The listing builds one solid part. Answer for the finished solid, in the listing's coordinates (mm). Round coordinates to 2 decimals unless told otherwise and drop trailing zeros. Write each loop counter-clockwise with the first axis right and the second up, starting at its lowest first coordinate (ties: lowest second). Pieces come first, ordered by that corner, then holes. Notation, with made-up numbers: (48, 79) - (59, 79) arc R23 cw to (59, 100) - close; hole circle Ø6 at (55, 46). An arc over 180 degrees is marked (long way). Return JSON: item names as keys, results as strings. Group by question number.
(1) Each of these flat-tipped pins is pushed along its axis until it touches: pin 1 (5 mm diameter, centred on x = -32.81, z = -52.81, fed in from -Y); pin 2 (3 mm diameter, centred on x = 33.5, z = 12.5, fed in from +Y); pin 3 (4 mm diameter, centred on x = 25, y = 575, fed in from +Z). Where does it stop, or does it pass through?
(2) Find the intervals of material crossed by line 1 along Y through (x, z) = (-1, -52.5); line 2 along Y through (x, z) = (-5, 2.5); line 3 along Z through (x, y) = (27.5, 52.5), in increasing order. Write a range as [from, to].
(3) Section A-A, the plane y = 30 is taken. Write down the section's boundary in (x, z), then the cut area to 3 significant figures.
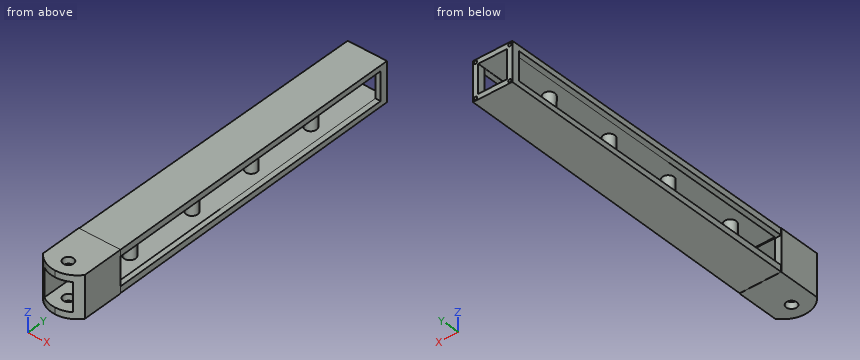
```python
from build123d import *

# Parameters (mm, degrees)
SKETCH1_W               = 80
SKETCH1_H               = 80
BOSS_EXTRUDE1_DEPTH     = 700
BOSS_EXTRUDE1_TAPER     = 0.2
SHELL2_T                = -10
SKETCH2_R               = 3
CUT_EXTRUDE1_DEPTH      = 10
CUT_EXTRUDE2_DEPTH      = 704.704483544
CUT_EXTRUDE2_DEPTH_BACK = 704.704483544
SKETCH4_W               = 55.112936398
SKETCH4_H               = 55.112936398
SKETCH8_W               = 80
SKETCH8_H               = 80
SKETCH8_W_2             = 55.112936398
SKETCH8_H_2             = 55.112936398
BOSS_EXTRUDE3_DEPTH     = 100
CUT_EXTRUDE4_DEPTH      = 706.691150691
CUT_EXTRUDE4_DEPTH_BACK = 706.691150691
SKETCH9_R               = 10
CUT_EXTRUDE5_DEPTH      = 706.691150691
CUT_EXTRUDE5_DEPTH_BACK = 706.691150691
CUT_EXTRUDE6_DEPTH      = 707.968504527
CUT_EXTRUDE6_DEPTH_BACK = 707.968504527
SKETCH13_W              = 54.721685152
SKETCH13_H              = 585.463174199
SKETCH14_R              = 11
BOSS_EXTRUDE4_DEPTH     = 68


with BuildPart() as part:
    # Sketch1 → Boss-Extrude1 (new body)
    with BuildSketch(Plane(origin=(0, 0, 0), x_dir=(1, 0, 0), z_dir=(0, 1, 0))):
        with Locations((0, 20)):
            Rectangle(SKETCH1_W, SKETCH1_H)
    extrude(amount=BOSS_EXTRUDE1_DEPTH, taper=BOSS_EXTRUDE1_TAPER)

    # Shell2
    shell2_openings = [part.faces().sort_by_distance(p)[0] for p in [
        (0, 700, -20),
    ]]
    offset(amount=SHELL2_T, openings=shell2_openings, kind=Kind.INTERSECTION)

    # Sketch2 → Cut-Extrude1 (cut)
    with BuildSketch(Plane(origin=(0, 700, 0), x_dir=(1, 0, 0), z_dir=(0, 1, 0))):
        with Locations(Location((-32.80796506, 52.80796506, 0), (0, 0, 270))):
            Circle(SKETCH2_R)
        with Locations(Location((32.80796506, 52.80796506, 0), (0, 0, 90))):
            Circle(SKETCH2_R)
        with Locations(Location((32.80796506, -12.80796506, 0), (0, 0, 270))):
            Circle(SKETCH2_R)
        with Locations(Location((-32.80796506, -12.80796506, 0), (0, 0, 90))):
            Circle(SKETCH2_R)
    extrude(amount=-CUT_EXTRUDE1_DEPTH, mode=Mode.SUBTRACT)

    # Sketch4 → Cut-Extrude2 (cut, two sides: drawn at the far end of the back side and taken through both)
    with BuildSketch(Plane(origin=(0, 700, 0), x_dir=(1, 0, 0), z_dir=(0, 1, 0)).offset(-CUT_EXTRUDE2_DEPTH_BACK)):
        with Locations((0, 20)):
            Rectangle(SKETCH4_W, SKETCH4_H)
    extrude(amount=CUT_EXTRUDE2_DEPTH + CUT_EXTRUDE2_DEPTH_BACK, mode=Mode.SUBTRACT)

    # Sketch8 → Boss-Extrude3 (add)
    with BuildSketch(Plane.XZ):
        with Locations((0, -20)):
            Rectangle(SKETCH8_W, SKETCH8_H)
        with Locations((0, -20)):
            Rectangle(SKETCH8_W_2, SKETCH8_H_2, mode=Mode.SUBTRACT)
    extrude(amount=-BOSS_EXTRUDE3_DEPTH)

    # Sketch9 → Cut-Extrude4 (cut, two sides: drawn at the far end of the back side and taken through both)
    with BuildSketch(Plane.XY.offset(20).offset(-CUT_EXTRUDE4_DEPTH_BACK)):
        with Locations((0, 30)):
            Circle(SKETCH9_R)
    extrude(amount=CUT_EXTRUDE4_DEPTH + CUT_EXTRUDE4_DEPTH_BACK, mode=Mode.SUBTRACT)

    # Sketch10 → Cut-Extrude5 (cut, two sides: drawn at the far end of the back side and taken through both)
    with BuildSketch(Plane.XY.offset(20).offset(-CUT_EXTRUDE5_DEPTH_BACK)):
        with BuildLine():
            Line((-40, 0), (-1.42e-07, 0))
            ThreePointArc((-1.42e-07, 0), (-22.333063671, 5.242902067), (-40, 19.876189785))
            Line((-40, 19.876189785), (-40, 0))
        make_face()
        with BuildLine():
            Line((-1.42e-07, 0), (40, 0))
            Line((40, 0), (40, 19.876189785))
            ThreePointArc((40, 19.876189785), (22.333063544, 5.242902004), (-1.42e-07, 0))
        make_face()
    extrude(amount=CUT_EXTRUDE5_DEPTH + CUT_EXTRUDE5_DEPTH_BACK, mode=Mode.SUBTRACT)

    # Sketch13 → Cut-Extrude6 (cut, two sides: drawn at the far end of the back side and taken through both)
    with BuildSketch(Plane(origin=(39.999512614, 0.139625206, 0), x_dir=(0, 0, -1), z_dir=(0.9999939076577905, 0.0034906514152237404, 0)).offset(-CUT_EXTRUDE6_DEPTH_BACK)):
        with Locations((20, 392.592570281)):
            Rectangle(SKETCH13_W, SKETCH13_H)
    extrude(amount=CUT_EXTRUDE6_DEPTH + CUT_EXTRUDE6_DEPTH_BACK, mode=Mode.SUBTRACT)

    # Sketch14 → Boss-Extrude4 (add)
    with BuildSketch(Plane(origin=(0, 0.209437809, -59.999268921), x_dir=(-1, 0, 0), z_dir=(0, 0.0034906514152237404, -0.9999939076577905))):
        with Locations(Location((0, 167.378380539, 0), (0, 0, 90))):
            Circle(SKETCH14_R)
        with Locations(Location((0, 306.630729062, 0), (0, 0, 90))):
            Circle(SKETCH14_R)
        with Locations(Location((0, 439.3151205, 0), (0, 0, 90))):
            Circle(SKETCH14_R)
        with Locations(Location((0, 573.229273125, 0), (0, 0, 90))):
            Circle(SKETCH14_R)
    extrude(amount=-BOSS_EXTRUDE4_DEPTH)


solid = part.part
```
Working result:
{
 "1": {"pin 1": "stops at y = 10.19", "pin 2": "stops at y = 690", "pin 3": "stops at z = 18"},
 "2": {"line 1": "y = [0.01, 20.05], [39.95, 700]", "line 2": "y = [157.57, 177.17], [296.83, 316.42], [429.51, 449.11], [563.43, 583.02]", "line 3": "z = [-60, -47.56], [7.56, 20]"},
 "3": {"outline": "(-40, -60) - (-10, -60) - (-10, -47.56) - (-27.56, -47.56) - (-27.56, 7.56) - (-10, 7.56) - (-10, 20) - (-40, 20) - close; (10, -60) - (40, -60) - (40, 20) - (10, 20) - (10, 7.56) - (27.56, 7.56) - (27.56, -47.56) - (10, -47.56) - close", "area": "2,860 mm^2"}
}
